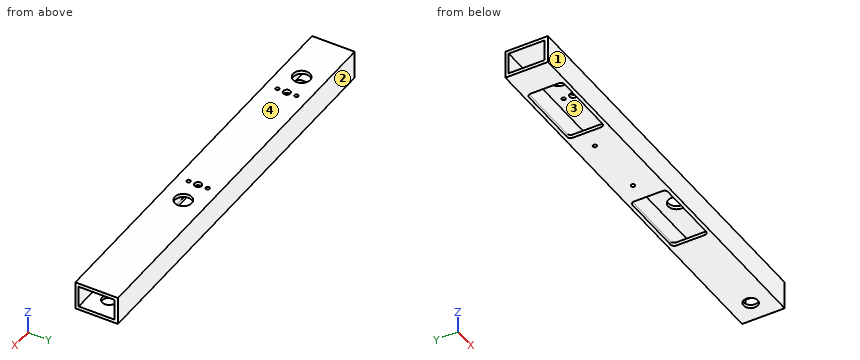
```python
from build123d import *

# Parameters (mm, degrees)
SKETCH1_W                = 25.4
SKETCH1_H                = 38.1
SKETCH1_W_2              = 19.304
SKETCH1_H_2              = 32.004
BOSS_EXTRUDE1_DEPTH      = 355.6
CUT_EXTRUDE1_REACH       = 27.4
SKETCH2_R                = 6.35
CUT_EXTRUDE4_REACH       = 27.4
SKETCH5_R                = 7.62
CUT_EXTRUDE5_REACH       = 27.4
SKETCH6_R                = 3.175
CUT_EXTRUDE6_REACH       = 27.4
M3_CLEARANCE_HOLE1_D     = 3.4
M3_CLEARANCE_HOLE1_DEPTH = 3.048
M3_CLEARANCE_HOLE2_D     = 3.4
M3_CLEARANCE_HOLE2_DEPTH = 3.048


with BuildPart() as part:
    # Sketch1 → Boss-Extrude1 (new body)
    with BuildSketch(Plane(origin=(0, 0, 0), x_dir=(0, 0, -1), z_dir=(1, 0, 0))):
        Rectangle(SKETCH1_W, SKETCH1_H)
        Rectangle(SKETCH1_W_2, SKETCH1_H_2, mode=Mode.SUBTRACT)
    extrude(amount=BOSS_EXTRUDE1_DEPTH)

    # Sketch2 → Cut-Extrude1 (cut, up to next)
    with BuildSketch(Plane(origin=(0, 0, -12.7), x_dir=(-1, 0, 0), z_dir=(0, 0, -1)), mode=Mode.PRIVATE) as cut_extrude1_sk1:
        with Locations((-336.55, 0)):
            Circle(SKETCH2_R)
    cut_extrude1_tool1 = extrude(cut_extrude1_sk1.sketch, amount=-CUT_EXTRUDE1_REACH, mode=Mode.PRIVATE) & part.part
    add(cut_extrude1_tool1.solids().sort_by_distance((336.55, 0, -12.7))[0], mode=Mode.SUBTRACT)

    # Sketch5 → Cut-Extrude4 (cut, up to next)
    with BuildSketch(Plane.XY.offset(12.7), mode=Mode.PRIVATE) as cut_extrude4_sk1:
        with Locations((47.625, 0)):
            Circle(SKETCH5_R)
    cut_extrude4_tool1 = extrude(cut_extrude4_sk1.sketch, amount=-CUT_EXTRUDE4_REACH, mode=Mode.PRIVATE) & part.part
    add(cut_extrude4_tool1.solids().sort_by_distance((47.625, 0, 12.7))[0], mode=Mode.SUBTRACT)
    # Sketch5 → Cut-Extrude4 (cut, up to next)
    with BuildSketch(Plane.XY.offset(12.7), mode=Mode.PRIVATE) as cut_extrude4_sk2:
        with Locations((225.425, 0)):
            Circle(SKETCH5_R)
    cut_extrude4_tool2 = extrude(cut_extrude4_sk2.sketch, amount=-CUT_EXTRUDE4_REACH, mode=Mode.PRIVATE) & part.part
    add(cut_extrude4_tool2.solids().sort_by_distance((225.425, 0, 12.7))[0], mode=Mode.SUBTRACT)

    # Sketch6 → Cut-Extrude5 (cut, up to next)
    with BuildSketch(Plane.XY.offset(12.7), mode=Mode.PRIVATE) as cut_extrude5_sk1:
        with Locations((69.85, 0)):
            Circle(SKETCH6_R)
    cut_extrude5_tool1 = extrude(cut_extrude5_sk1.sketch, amount=-CUT_EXTRUDE5_REACH, mode=Mode.PRIVATE) & part.part
    add(cut_extrude5_tool1.solids().sort_by_distance((69.85, 0, 12.7))[0], mode=Mode.SUBTRACT)
    # Sketch6 → Cut-Extrude5 (cut, up to next)
    with BuildSketch(Plane.XY.offset(12.7), mode=Mode.PRIVATE) as cut_extrude5_sk2:
        with Locations((203.2, 0)):
            Circle(SKETCH6_R)
    cut_extrude5_tool2 = extrude(cut_extrude5_sk2.sketch, amount=-CUT_EXTRUDE5_REACH, mode=Mode.PRIVATE) & part.part
    add(cut_extrude5_tool2.solids().sort_by_distance((203.2, 0, 12.7))[0], mode=Mode.SUBTRACT)

    # Sketch7 → Cut-Extrude6 (cut, up to next)
    with BuildSketch(Plane(origin=(0, 0, -12.7), x_dir=(-1, 0, 0), z_dir=(0, 0, -1)), mode=Mode.PRIVATE) as cut_extrude6_sk1:
        with BuildLine():
            Line((-242.8875, -15.875), (-185.7375, -15.875))
            ThreePointArc((-185.7375, -15.875), (-183.49243597, -14.94506403), (-182.5625, -12.7))
            Line((-182.5625, -12.7), (-182.5625, 12.7))
            ThreePointArc((-182.5625, 12.7), (-183.49243597, 14.94506403), (-185.7375, 15.875))
            Line((-185.7375, 15.875), (-242.8875, 15.875))
            ThreePointArc((-242.8875, 15.875), (-245.13256403, 14.94506403), (-246.0625, 12.7))
            Line((-246.0625, 12.7), (-246.0625, -12.7))
            ThreePointArc((-246.0625, -12.7), (-245.13256403, -14.94506403), (-242.8875, -15.875))
        make_face()
    cut_extrude6_tool1 = extrude(cut_extrude6_sk1.sketch, amount=-CUT_EXTRUDE6_REACH, mode=Mode.PRIVATE) & part.part
    add(cut_extrude6_tool1.solids().sort_by_distance((214.3125, 0, -12.7))[0], mode=Mode.SUBTRACT)
    # Sketch7 → Cut-Extrude6 (cut, up to next)
    with BuildSketch(Plane(origin=(0, 0, -12.7), x_dir=(-1, 0, 0), z_dir=(0, 0, -1)), mode=Mode.PRIVATE) as cut_extrude6_sk2:
        with BuildLine():
            Line((-87.3125, -15.875), (-30.1625, -15.875))
            ThreePointArc((-30.1625, -15.875), (-27.91743597, -14.94506403), (-26.9875, -12.7))
            Line((-26.9875, -12.7), (-26.9875, 12.7))
            ThreePointArc((-26.9875, 12.7), (-27.91743597, 14.94506403), (-30.1625, 15.875))
            Line((-30.1625, 15.875), (-87.3125, 15.875))
            ThreePointArc((-87.3125, 15.875), (-89.55756403, 14.94506403), (-90.4875, 12.7))
            Line((-90.4875, 12.7), (-90.4875, -12.7))
            ThreePointArc((-90.4875, -12.7), (-89.55756403, -14.94506403), (-87.3125, -15.875))
        make_face()
    cut_extrude6_tool2 = extrude(cut_extrude6_sk2.sketch, amount=-CUT_EXTRUDE6_REACH, mode=Mode.PRIVATE) & part.part
    add(cut_extrude6_tool2.solids().sort_by_distance((58.7375, 0, -12.7))[0], mode=Mode.SUBTRACT)

    # M3 Clearance Hole1
    with Locations(Plane(origin=(165.1, 3.175, -12.7), x_dir=(-1, 0, 0), z_dir=(0, 0, -1))):
        with Locations((0, 0), (57.15, 0)):
            Hole(M3_CLEARANCE_HOLE1_D / 2, depth=M3_CLEARANCE_HOLE1_DEPTH)

    # M3 Clearance Hole2
    with Locations(Plane(origin=(69.85, 8.5, 12.7), x_dir=(1, 0, 0), z_dir=(0, 0, 1))):
        with Locations((0, 0), (0, -17), (133.35, 0), (133.35, -17)):
            Hole(M3_CLEARANCE_HOLE2_D / 2, depth=M3_CLEARANCE_HOLE2_DEPTH)


solid = part.part
```
Part model, mm, in its own coordinate system. Face numbers are marked on the shaded views. Give positions to 0.01 mm unless a question says otherwise; leave off trailing zeros. Order: outer loops, then holes, each group sorted by start corner. A loop starts at its lowest first (then second) coordinate and runs counter-clockwise, first axis right, second up. Notation, with made-up numbers: (16.25, 72) - (55.25, 72) arc R25 cw to (55.25, 96) - close; hole circle Ø6 at (33.5, 82). An arc over 180 degrees is marked (long way). Use one line per item in the form item = value.
Item 1: Two-plate mould, pull along Y, no slides. Class the marked faces 1, 2, 3 and 4: released by +Y, released by -Y, zero draft, split by the parting line, or undercut.
Solution:
face_1 = released by -Y
face_2 = released by +Y
face_3 = undercut
face_4 = zero draft
Item 2: Pin check, flat tips, straight feed: pin 1 Ø2.5 at (x, y) = (69.85, -8.5) entering from +Z; pin 2 Ø5.5 at (x, y) = (69.85, 8.5) entering from -Z. Stop position of each tip, or through.
Solution:
pin_1 = through
pin_2 = 9.65
Item 3: Slice it at C-C on x = 336.55. Give the cut face in (y, z).
Solution:
outline = (-19.05, -12.7) - (-6.35, -12.7) - (-6.35, -9.65) - (-16, -9.65) - (-16, 9.65) - (16, 9.65) - (16, -9.65) - (6.35, -9.65) - (6.35, -12.7) - (19.05, -12.7) - (19.05, 12.7) - (-19.05, 12.7) - close
Item 4: Slice it at B-B on z = -4.5. Give the cut face in (x, y), and give its area (3 significant figures).
Solution:
outline = (0, -19.05) - (355.6, -19.05) - (355.6, -16) - (0, -16) - close; (0, 16) - (355.6, 16) - (355.6, 19.05) - (0, 19.05) - close
area = 2,170 mm2
Item 5: Slice it at A-A on x = 254. Give the cut face in (y, z), and give its area (3 significant figures).
Solution:
outline = (-19.05, -12.7) - (19.05, -12.7) - (19.05, 12.7) - (-19.05, 12.7) - close; hole (-16, -9.65) - (16, -9.65) - (16, 9.65) - (-16, 9.65) - close
area = 350 mm2
Item 6: Probe probe 1 along Y at (x, z) = (69.85, 10.65) (3 decimals); probe 2 along X at (y, z) = (7.5, -10); probe 3 along Y at (x, z) = (38, -5.75). List the from-to ranges inside material, lowest first. Write a range as from..to.
Solution:
probe_1 = -19.05..-10.2, -6.8..-3.175, 3.175..6.8, 10.2..19.05
probe_2 = 0..26.99, 90.49..182.56, 246.06..355.6
probe_3 = -19.05..-16, 16..19.05
